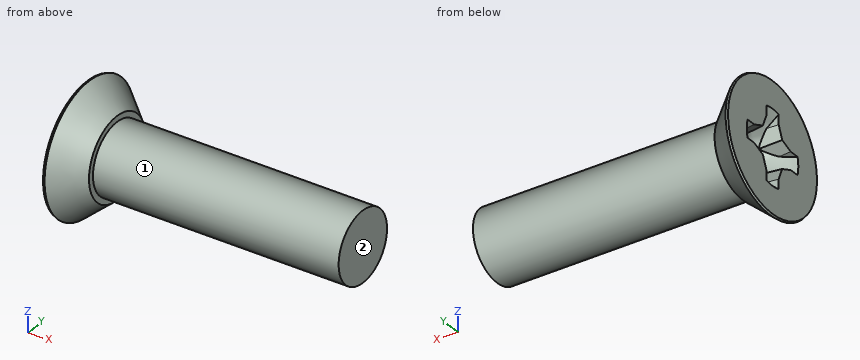
from build123d import *

# Parameters (mm, degrees)
CUT_EXTRUDE1_REACH = 22.129
CIRPATTERN1_COUNT  = 4
DRAFT1_ANGLE       = 5
CHAMFER1_SIZE      = 0.183896
CHAMFER1_SIZE2     = 0.168435197


with BuildPart() as part:
    # Sketch2 → Revolve1 (revolve)
    with BuildSketch(Plane.XY, mode=Mode.PRIVATE) as revolve1_sk:
        Polygon((-9.525, 0), (9.525, 0), (9.525, 2.413), (-7.4676, 2.413), (-7.4676, 2.808929466), (-9.525, 4.5974), align=None)
    revolve(revolve1_sk.sketch.rotate(Axis((-9.525, 0, 0), (1, 0, 0)), 180), axis=Axis((-9.525, 0, 0), (1, 0, 0)))

    # Cut-Extrude1: up to this cone (the profile starts inside it)
    cut_extrude1_end = Plane(origin=(-9.525, 0, 0), z_dir=(-1, 0, 0)).offset(-2.952835668) * Cone(1e-06, 24.469290226, 28.148697423, align=(Align.CENTER, Align.CENTER, Align.MIN), mode=Mode.PRIVATE)
    # Sketch3 → Cut-Extrude1 (cut, up to the surface)
    with BuildSketch(Plane.ZY.offset(9.525), mode=Mode.PRIVATE) as cut_extrude1_sk1:
        with BuildLine():
            Line((0, 0), (3.064933333, 0))
            ThreePointArc((3.064933333, 0), (3.04941298, 0.308053268), (3.003009105, 0.612986667))
            Line((3.003009105, 0.612986667), (1.807997886, 0.612986667))
            Line((1.807997886, 0.612986667), (0.962997349, 0.962997349))
            Line((0.962997349, 0.962997349), (0.612986667, 1.807997886))
            Line((0.612986667, 1.807997886), (0.612986667, 3.003009105))
            ThreePointArc((0.612986667, 3.003009105), (0.308053268, 3.04941298), (0, 3.064933333))
            Line((0, 3.064933333), (0, 0))
        make_face()
    cut_extrude1_tool1 = extrude(cut_extrude1_sk1.sketch, amount=-CUT_EXTRUDE1_REACH, mode=Mode.PRIVATE) & cut_extrude1_end
    cut_extrude1 = cut_extrude1_tool1.solids().sort_by_distance((-9.525, 1.532467, 0.043345))[0]
    add(cut_extrude1, mode=Mode.SUBTRACT)

    # CirPattern1: Cut-Extrude1 ×4 about axis
    cirpattern1_axis = Axis((0, 0, 0), (1, 0, 0))
    for i in range(1, CIRPATTERN1_COUNT):
        add(cut_extrude1.rotate(cirpattern1_axis, i * 360 / CIRPATTERN1_COUNT), mode=Mode.SUBTRACT)

    # Draft1
    draft1_faces = [part.faces().sort_by_distance(p)[0] for p in [
        (-9.272207982, 0.612986667, -2.036620878),
        (-8.957922731, 0.804804583, -1.344908471),
        (-8.957922731, 1.344908471, -0.804804583),
        (-9.272207982, 2.036620878, -0.612986667),
        (-9.272207982, 2.036620878, 0.612986667),
        (-8.957922731, 1.344908471, 0.804804583),
        (-8.957922731, 0.804804583, 1.344908471),
        (-9.272207982, 0.612986667, 2.036620878),
        (-9.272207982, -0.612986667, 2.036620878),
        (-8.957922731, -0.804804583, 1.344908471),
        (-8.957922731, -1.344908471, 0.804804583),
        (-9.272207982, -2.036620878, 0.612986667),
        (-9.272207982, -2.036620878, -0.612986667),
        (-8.957922731, -1.344908471, -0.804804583),
        (-8.957922731, -0.804804583, -1.344908471),
        (-9.272207982, -0.612986667, -2.036620878),
    ]]
    draft(draft1_faces, Plane(origin=(-9.525, 0, 0), x_dir=(0, -1, 0), z_dir=(-1, 0, 0)), DRAFT1_ANGLE)

    # Chamfer1
    chamfer1_edges = [part.edges().sort_by_distance(p)[0] for p in [
        (-9.525, 4.5974, 0),
    ]]
    chamfer1_side = [part.faces().sort_by_distance(p)[0] for p in [
        (-8.4963, 3.703164733, 0),
    ]]
    chamfer(chamfer1_edges, length=CHAMFER1_SIZE, length2=CHAMFER1_SIZE2, reference=chamfer1_side[0])


solid = part.part
The model under review builds one solid part; all positions refer to its coordinate system, in mm. Face numbers are marked on the shaded views. A direction names the side the tool comes from. Round coordinates to 2 decimals unless told otherwise and drop trailing zeros. Write each loop counter-clockwise with the first axis right and the second up, starting at its lowest first coordinate (ties: lowest second). Pieces come first, ordered by that corner, then holes. Notation, with made-up numbers: (80, -8) -> (91, -8) arc R19 ccw to (91, 28) -> close; hole circle Ø11 at (-17, 45.5). An arc over 180 degrees is marked (long way). Answer as a JSON object with one key per item and string values.
1. To check wall thickness, follow line 1 along X through (y, z) = (0, 2.75) (3 decimals); line 2 along Y through (x, z) = (6.5, -1.5); line 3 along Y through (x, z) = (-2, -0.25). State the ranges of each line that lie inside material, in increasing order.
Results found:
{"line 1": "x = -9.525 to -7.468", "line 2": "y = -1.89 to 1.89", "line 3": "y = -2.4 to 2.4"}
2. Clearance check with flat-ended pins moving along their axes: pin 1 (3 mm diameter, centred on x = 3.5, y = -1.5, fed in from +Z); pin 2 (2 mm diameter, centred on x = 6, y = 0.5, fed in from -Z). State where each tip first meets the part, or that it passes through.
Results found:
{"pin 1": "stops at z = 2.41", "pin 2": "stops at z = -2.41"}
3. We need section A-A on x = 0.75. State the section outline as (y, z) points.
Results found:
{"outline": "circle Ø4.83 at (0, 0)"}
4. Machinability: for the marked faces 1 and 2, which of the approach directions +Z, -Z, +X, -X, +Y, -Y give a long, thin tool a straight path to every point of the face, cutting with its end or side? Answer none if there is none.
Results found:
{"face 1": "+X", "face 2": "+Z, -Z, +X, +Y, -Y"}
